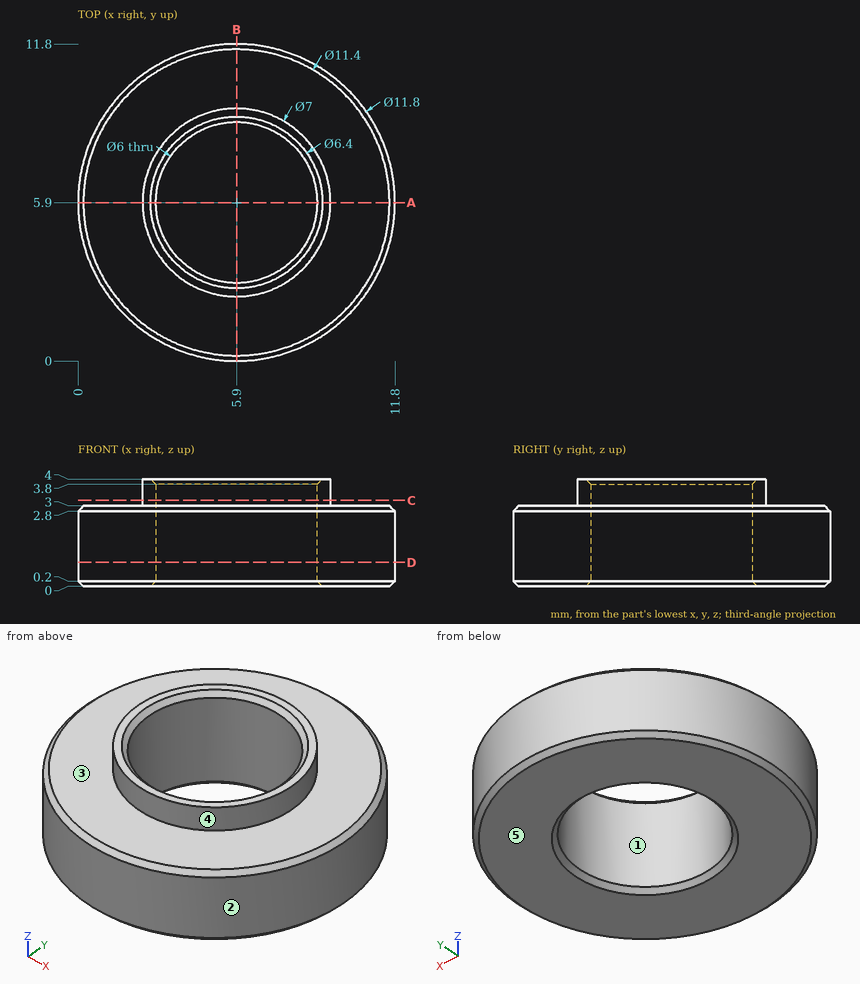
Study the drawing (mm; zero at the part's minimum x, y, z) and answer. A direction names the side the tool comes from. Coordinates: 2 decimals unless noted, no trailing zeros. Write each loop counter-clockwise with the first axis right and the second up, starting at its lowest first coordinate (ties: lowest second). Pieces come first, ordered by that corner, then holes. Notation, with made-up numbers: (78.25, 47) - (99.25, 47) arc R21 ccw to (99.25, 82) - close; hole circle Ø9 at (88.5, 2). An arc over 180 degrees is marked (long way). One line per item, written item: value.
1) For a pull along X with two mould halves and no side action, classify the marked faces 1, 2 and 3 as pulls with the +X half, pulls with the -X half, needs draft (parallel to the pull), parting line crosses it, or undercut.
Geometry check:
face 1: undercut
face 2: parting line crosses it
face 3: needs draft
2) Find section D-D (z = 0.9). Give the vertices of the cut face in (x, y).
Geometry check:
outline: circle Ø11.8 at (5.9, 5.9); hole circle Ø6 at (5.9, 5.9)
3) A tool of negligible diameter and unlimited length cuts with its end or side. For the marked faces 4 and 5, from which of +Z, -Z, +X, -X, +Y, -Y can it reach the whole face along a straight path? Write none if from no direction.
Geometry check:
face 4: +Z
face 5: -Z, +X, -X, +Y, -Y
4) Consider line 1 along Y through (x, z) = (5.9, 1.3); line 2 along Z through (x, y) = (1, 4). Determine where each line is inside the solid, lowest interval first. Write a range as from..to.
Geometry check:
line 1: y = 0..2.9, 8.9..11.8
line 2: z = 0..3
5) Find section C-C (z = 3.2). Give the vertices of the cut face in (x, y).
Geometry check:
outline: circle Ø7 at (5.9, 5.9); hole circle Ø6 at (5.9, 5.9)
6) Find section A-A (y = 5.9). Give the vertices of the cut face in (x, z).
Geometry check:
outline: (0, 0.2) - (0.2, 0) - (2.7, 0) - (2.9, 0.2) - (2.9, 3.8) - (2.7, 4) - (2.4, 4) - (2.4, 3) - (0.2, 3) - (0, 2.8) - close; (8.9, 0.2) - (9.1, 0) - (11.6, 0) - (11.8, 0.2) - (11.8, 2.8) - (11.6, 3) - (9.4, 3) - (9.4, 4) - (9.1, 4) - (8.9, 3.8) - close
